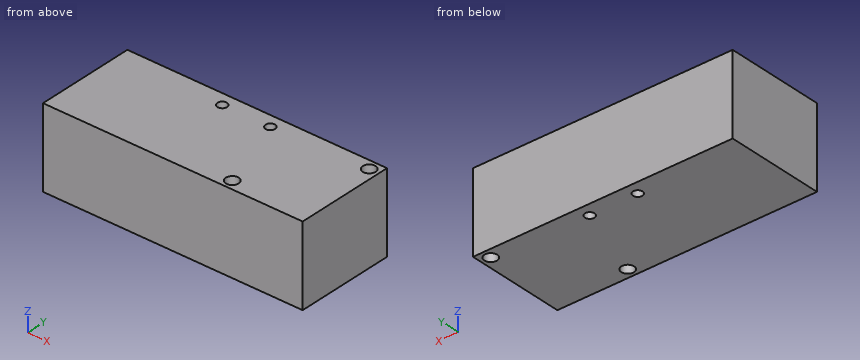
Autodesk Inventor part; units mm, degrees
ref_plane "YZ Plane" through (0, 0, 0) normal (1, 0, 0) x (0, 1, 0)
ref_plane "XZ Plane" through (0, 0, 0) normal (0, 1, 0) x (-1, 0, 0)
ref_plane "XY Plane" through (0, 0, 0) normal (0, 0, 1) x (1, 0, 0)
sketch "Sketch1" plane through (0, 0, 0) normal (0, 0, 1) x (1, 0, 0)
  line L0 (-40.5, -15.5) -> (40.5, -15.5)
  line L1 (40.5, -15.5) -> (40.5, 15.5)
  line L2 (40.5, 15.5) -> (-40.5, 15.5)
  line L3 (-40.5, 15.5) -> (-40.5, -15.5)
  line L4 (-40.5, -15.5) -> (40.5, 15.5) construction
  line L5 (40.5, -15.5) -> (-40.5, 15.5) construction
  line L6 (37.5, 15.5) -> (37.5, -15.5)
  circle A0 centre (37.5, 12.5) radius 2
  line L7 (16, -15.5) -> (16, 15.5)
  circle A1 centre (16, -12.5) radius 2
  line L8 (7.5, -15.5) -> (7.5, 15.5)
  circle A2 centre (7.5, 11.5) radius 1.5
  line L9 (-7.5, -15.5) -> (-7.5, 15.5)
  circle A3 centre (-7.5, 11.5) radius 1.5
  point P0 (0, 0)
  dimension "d0" = 3
  dimension "d1" = 81
  dimension "d2" = 31
  dimension "d3" = 4
  dimension "d4" = 3
  dimension "d5" = 24.5
  dimension "d6" = 4
  dimension "d7" = 3
  dimension "d8" = 30
  dimension "d9" = 3
  dimension "d11" = 4
  dimension "d12" = 15
  dimension "d13" = 3
extrude "Extrusion1" add sketch "Sketch1" along normal blind 25 contours L3 L2 L9 A3 L0 | L9 A3 L2 L8 A2 L0 | L8 A2 L2 L7 A1 L0 | L7 A1 L2 L6 A0 L0 | L6 A0 L2 L1 L0
properties part number "Bluepill" material "Silver"
Source: CAD feature listing. Evaluate the final solid. Frame: model axes, mm. Give positions to 0.01 mm unless a question says otherwise; leave off trailing zeros. Loops run counter-clockwise (first coordinate to the right, second up) from the corner with the lowest first, then second, coordinate; pieces in that order, holes last. Notation, with made-up numbers: (-21, -14.75) -> (33, -14.75) arc R22 ccw to (33, 11.25) -> close; hole circle Ø7 at (-40, 18). An arc over 180 degrees is marked (long way). Use a Markdown table: item, result. Add a question column.
1) First-contact query: pin 1 (5 mm diameter, centred on x = 16, y = -12.5, fed in from -Z). Flat tip, straight axial feed; report the tip coordinate or a pass-through.
2) Section query A-A, the plane x = -7.5. Return the cut outline in (y, z).
3) Section query D-D, the plane x = 16. Return the cut outline in (y, z).
4) Line query: line 1 along Y through (x, z) = (16, 19.5); line 2 along X through (y, z) = (-12.5, 7.75); line 3 along Y through (x, z) = (-7.5, 10.5). Output: solid intervals per line, ascending. Write a range as [from, to].
5) Section query C-C, the plane y = 11.5. Return the cut outline in (x, z), then the cut area to 3 significant figures.
6) Section query B-B, the plane z = 20.5. Return the cut outline in (x, y), then the cut area to 3 significant figures.
Numbers:
| question | item | result |
|---|---|---|
| 1 | pin 1 | stops at z = 0 |
| 2 | outline | (-15.5, 0) -> (10, 0) -> (10, 25) -> (-15.5, 25) -> close; (13, 0) -> (15.5, 0) -> (15.5, 25) -> (13, 25) -> close |
| 3 | outline | (-15.5, 0) -> (-14.5, 0) -> (-14.5, 25) -> (-15.5, 25) -> close; (-10.5, 0) -> (15.5, 0) -> (15.5, 25) -> (-10.5, 25) -> close |
| 4 | line 1 | y = [-15.5, -14.5], [-10.5, 15.5] |
| 4 | line 2 | x = [-40.5, 14], [18, 40.5] |
| 4 | line 3 | y = [-15.5, 10], [13, 15.5] |
| 5 | outline | (-40.5, 0) -> (-9, 0) -> (-9, 25) -> (-40.5, 25) -> close; (-6, 0) -> (6, 0) -> (6, 25) -> (-6, 25) -> close; (9, 0) -> (35.77, 0) -> (35.77, 25) -> (9, 25) -> close; (39.23, 0) -> (40.5, 0) -> (40.5, 25) -> (39.23, 25) -> close |
| 5 | area | 1,790 mm2 |
| 6 | outline | (-40.5, -15.5) -> (40.5, -15.5) -> (40.5, 15.5) -> (-40.5, 15.5) -> close; hole circle Ø3 at (-7.5, 11.5); hole circle Ø3 at (7.5, 11.5); hole circle Ø4 at (16, -12.5); hole circle Ø4 at (37.5, 12.5) |
| 6 | area | 2,470 mm2 |
